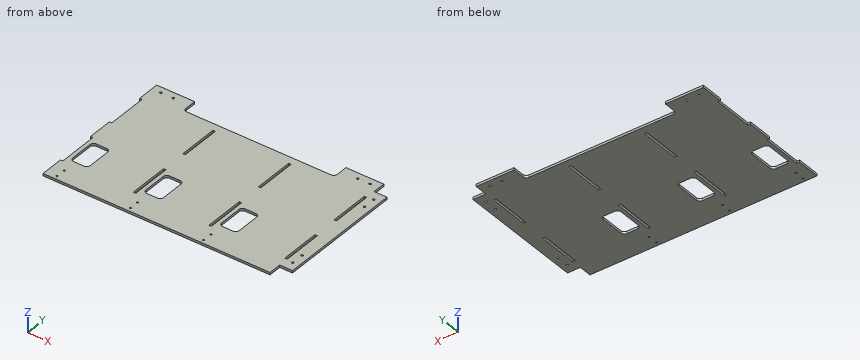
```python
from build123d import *

# Parameters (mm, degrees)
SKETCH_1_W          = 500.8
SKETCH_1_H          = 300.8
EXTRUDE_1_DEPTH     = 4.75
SKETCH_2_W          = 25.4
SKETCH_2_H          = 25.4
SKETCH_2_W_2        = 4.75
SKETCH_2_H_2        = 80
CUT_EXTRUDE_1_DEPTH = 25.4
SKETCH_3_R          = 2.15
SKETCH_3_R_2        = 2.150000004
CUT_EXTRUDE_2_DEPTH = 5
SKETCH_5_W          = 35
SKETCH_5_H          = 60
SKETCH_5_W_2        = 300
SKETCH_5_H_2        = 30
CUT_EXTRUDE_3_DEPTH = 10
FILLET_1_R          = 7
SKETCH_6_R          = 1.75
CUT_EXTRUDE_4_DEPTH = 10


with BuildPart() as part:
    # 草圖1 → 填料-伸長1 (new body)
    with BuildSketch(Plane.XY):
        Rectangle(SKETCH_1_W, SKETCH_1_H)
    extrude(amount=EXTRUDE_1_DEPTH)

    # 草圖2 → 除料-伸長1 (cut)
    with BuildSketch(Plane(origin=(0, 0, 0), x_dir=(-1, 0, 0), z_dir=(0, 0, -1))):
        with Locations((-237.7, 137.7)):
            Rectangle(SKETCH_2_W, SKETCH_2_H)
        with Locations((-237.7, -137.7)):
            Rectangle(SKETCH_2_W, SKETCH_2_H)
        Polygon((250.4, -150.4), (250.4, 150.4), (225, 150.4), (225, 105.4), (220.25, 105.4), (220.25, 25.4), (225, 25.4), (225, -24.4), (220.25, -24.4), (220.25, -104.4), (225, -104.4), (225, -150.4), align=None)
        with Locations((-222.625, 65.4)):
            Rectangle(SKETCH_2_W_2, SKETCH_2_H_2)
        with Locations((-222.625, -65.4)):
            Rectangle(SKETCH_2_W_2, SKETCH_2_H_2)
        with Locations((-72.625, 65.4)):
            Rectangle(SKETCH_2_W_2, SKETCH_2_H_2)
        with Locations((77.375, 65.4)):
            Rectangle(SKETCH_2_W_2, SKETCH_2_H_2)
        with Locations((77.375, -65.4)):
            Rectangle(SKETCH_2_W_2, SKETCH_2_H_2)
        with Locations((-72.625, -65.4)):
            Rectangle(SKETCH_2_W_2, SKETCH_2_H_2)
    extrude(amount=-CUT_EXTRUDE_1_DEPTH, mode=Mode.SUBTRACT)

    # 草圖3 → 除料-伸長2 (cut)
    with BuildSketch(Plane.XY.offset(4.75)):
        with Locations((-207.3, 137.7)):
            Circle(SKETCH_3_R)
        with Locations((-182.8, 137.7)):
            Circle(SKETCH_3_R)
        with Locations((182.8, 137.7)):
            Circle(SKETCH_3_R)
        with Locations((207.3, 137.7)):
            Circle(SKETCH_3_R)
        with Locations((237.7, 107.3)):
            Circle(SKETCH_3_R)
        with Locations((237.7, 82.8)):
            Circle(SKETCH_3_R)
        with Locations((237.7, -82.800000014)):
            Circle(SKETCH_3_R_2)
        with Locations((237.7, -107.300000014)):
            Circle(SKETCH_3_R_2)
        with Locations((-237.7, 107.3)):
            Circle(SKETCH_3_R)
        with Locations((-237.7, 82.8)):
            Circle(SKETCH_3_R)
        with Locations((-237.7, -82.800000014)):
            Circle(SKETCH_3_R_2)
        with Locations((-237.7, -107.300000014)):
            Circle(SKETCH_3_R_2)
    extrude(amount=-CUT_EXTRUDE_2_DEPTH, mode=Mode.SUBTRACT)

    # 草圖5 → 除料-伸長3 (cut)
    with BuildSketch(Plane.XY.offset(4.75)):
        with Locations((100, -65.4)):
            Rectangle(SKETCH_5_W, SKETCH_5_H)
        with Locations((-50, -65.4)):
            Rectangle(SKETCH_5_W, SKETCH_5_H)
        with Locations((-195.25, -65.4)):
            Rectangle(SKETCH_5_W, SKETCH_5_H)
        with Locations((0, 135.4)):
            Rectangle(SKETCH_5_W_2, SKETCH_5_H_2)
    extrude(amount=-CUT_EXTRUDE_3_DEPTH, mode=Mode.SUBTRACT)

    # 圓角1
    fillet_1_edges = [part.edges().sort_by_distance(p)[0] for p in [
        (-150, 120.4, 2.375),
        (150, 120.4, 2.375),
        (-177.75, -35.4, 2.375),
        (-177.75, -95.4, 2.375),
        (-212.75, -95.4, 2.375),
        (-212.75, -35.4, 2.375),
        (-32.5, -35.4, 2.375),
        (-32.5, -95.4, 2.375),
        (-67.5, -95.4, 2.375),
        (-67.5, -35.4, 2.375),
        (117.5, -35.4, 2.375),
        (117.5, -95.4, 2.375),
        (82.5, -95.4, 2.375),
        (82.5, -35.4, 2.375),
    ]]
    fillet(fillet_1_edges, radius=FILLET_1_R)

    # 草圖6 → 除料-伸長4 (cut)
    with BuildSketch(Plane.XY.offset(4.75)):
        with Locations((-202.75, -142.9)):
            Circle(SKETCH_6_R)
        with Locations((-202.75, -123.9)):
            Circle(SKETCH_6_R)
        with Locations((-57.5, -142.9)):
            Circle(SKETCH_6_R)
        with Locations((-57.5, -123.9)):
            Circle(SKETCH_6_R)
        with Locations((87.75, -142.9)):
            Circle(SKETCH_6_R)
        with Locations((87.75, -123.9)):
            Circle(SKETCH_6_R)
    extrude(amount=-CUT_EXTRUDE_4_DEPTH, mode=Mode.SUBTRACT)


solid = part.part
```
Model file for the job. Use its own axes, mm. Give positions to 0.01 mm unless a question says otherwise; leave off trailing zeros. Loops run counter-clockwise (first coordinate to the right, second up) from the corner with the lowest first, then second, coordinate; pieces in that order, holes last. Notation, with made-up numbers: (-25.75, -13) -> (-0.75, -13) arc R18 cw to (-0.75, -7) -> close; hole circle Ø9 at (34.5, -14). An arc over 180 degrees is marked (long way). Write each question's results on one line, items separated by ' | '.
(1) Cut at C-C on y = -130.5. List the corners of the cut face in (x, z).
Geometry results:
outline: (-225, 0) -> (225, 0) -> (225, 4.75) -> (-225, 4.75) -> close
(2) Flat gauge pins, fed straight in: pin 1 Ø1.4 at (x, z) = (-52.5, 3.5) entering from +Y; pin 2 Ø2 at (x, y) = (87.75, -123.9) entering from +Z; pin 3 Ø2 at (y, z) = (-31.5, 2) entering from -X. Where does each tip first touch, or does it go through?
Geometry results:
pin 1: stops at y = 120.4 | pin 2: passes through | pin 3: stops at x = -220.25
(3) Cut at B-B on z = 2.3. Give the number of separate pieces and of enclosed holes in the cut face, and give its area (3 significant figures).
Geometry results:
separate pieces: 1 | enclosed holes: 23 | area: 123,000 mm²
(4) Cut at A-A on x = -102. List the corners of the cut face in (y, z), and give its area (3 significant figures).
Geometry results:
outline: (-150.4, 0) -> (120.4, 0) -> (120.4, 4.75) -> (-150.4, 4.75) -> close | area: 1,290 mm²
(5) Probe line 1 along Y through (x, z) = (-57.5, 1.7); line 2 along X through (y, z) = (137.7, 1.8); line 3 along X through (y, z) = (77, 1.25). List the from-to ranges inside material, lowest first.
Geometry results:
line 1: y = -150.4 to -144.65, -141.15 to -125.65, -122.15 to -95.4, -35.4 to 120.4 | line 2: x = -225 to -209.45, -205.15 to -184.95, -180.65 to -150, 150 to 180.65, 184.95 to 205.15, 209.45 to 225 | line 3: x = -220.25 to -79.75, -75 to 70.25, 75 to 220.25, 225 to 250.4
